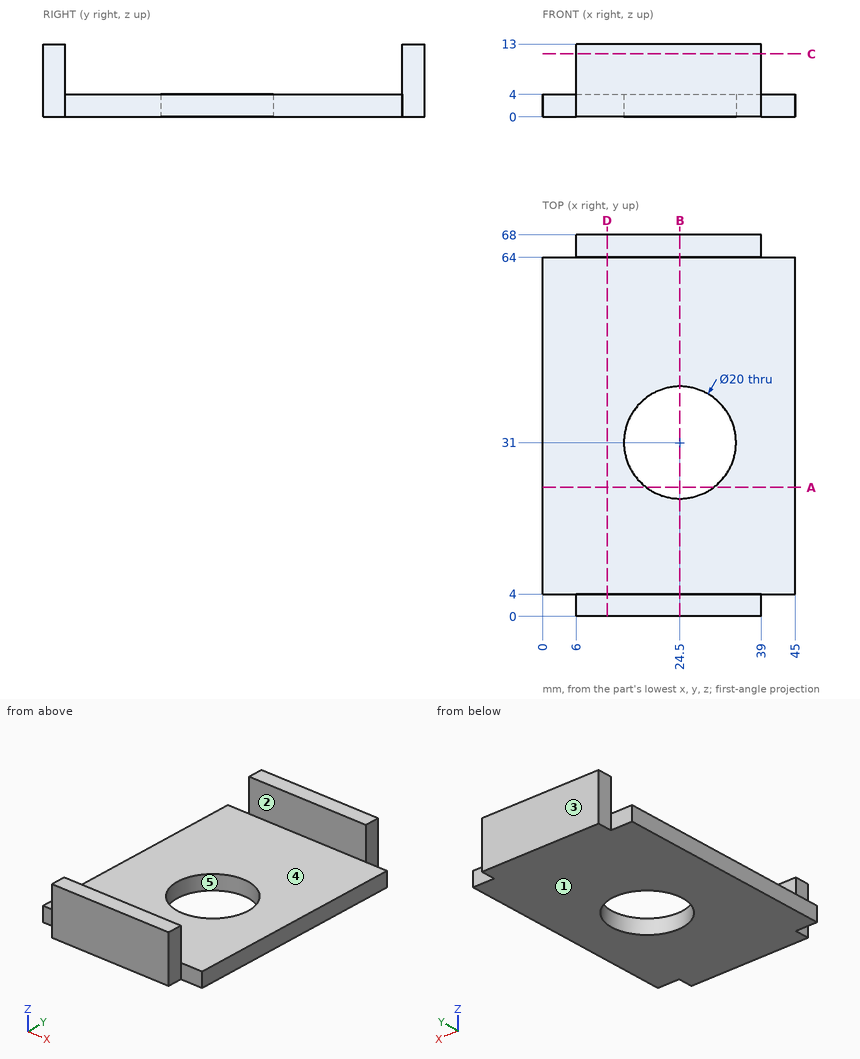
For this review, use the dimensioned drawing (mm, ordinates from the lowest corner) and the shaded views. A direction names the side the tool comes from. Coordinates: 2 decimals unless noted, no trailing zeros. Loops run counter-clockwise (first coordinate to the right, second up) from the corner with the lowest first, then second, coordinate; pieces in that order, holes last.
1. Add section D-D, the plane x = 11.5. Give the boundary of the cut face in (y, z).
2. For the marked faces 4 and 5, list the 3-axis set-ups (+Z, -Z, +X, -X, +Y, -Y) from which the entire face can be reached by the end or side of a thin tool; tool diameter is ignored.
3. Mouldability with a two-part tool opening along Y and no side actions: class the marked faces 1, 2 and 3 as +Y half, -Y half, draft (parallel to the pull), parting line (faces both ways), or undercut.
4. Add section C-C, the plane z = 11.25. Give the boundary of the cut face in (x, y).
5. Insertion check: P1, Ø1.2, axis at x = 43.5, z = 2.5, coming from the +Y side; P2, Ø23, axis at x = 24.5, y = 31, coming from the +Z side; P3, Ø1.2, axis at y = 1.5, z = 8.5, coming from the +X side. Each pin has a flat end and moves straight along its axis. Give the tip position at first contact, or say it passes through.
6. For line 1 (Y direction, x = 24.5, z = 2.45); line 2 (Y direction, x = 34.5, z = 11); line 3 (Z direction, x = 5, y = 12), list the stretches that pass through material, from the lowest coordinate up.
7. Add section A-A, the plane y = 23. Give the boundary of the cut face in (x, z).
8. Add section B-B, the plane x = 24.5. Give the boundary of the cut face in (y, z).
Result:
1. outline: (0, 0) - (68, 0) - (68, 13) - (64, 13) - (64, 4) - (4, 4) - (4, 13) - (0, 13) - close
2. face 4: +Z, +X, -X
2. face 5: +Z, -Z
3. face 1: draft
3. face 2: undercut
3. face 3: +Y half
4. outline: (6, 0) - (39, 0) - (39, 4) - (6, 4) - close; (6, 64) - (39, 64) - (39, 68) - (6, 68) - close
5. P1: stops at y = 64
5. P2: stops at z = 4
5. P3: stops at x = 39
6. line 1: y = 0 to 21, 41 to 68
6. line 2: y = 0 to 4, 64 to 68
6. line 3: z = 0 to 4
7. outline: (0, 0) - (18.5, 0) - (18.5, 4) - (0, 4) - close; (30.5, 0) - (45, 0) - (45, 4) - (30.5, 4) - close
8. outline: (0, 0) - (21, 0) - (21, 4) - (4, 4) - (4, 13) - (0, 13) - close; (41, 0) - (68, 0) - (68, 13) - (64, 13) - (64, 4) - (41, 4) - close
